Can you work these out from the model? Positions are in its coordinate system, mm. A direction names the side the tool comes from. Coordinates: 2 decimals unless noted, no trailing zeros. Order: outer loops, then holes, each group sorted by start corner. A loop starts at its lowest first (then second) coordinate and runs counter-clockwise, first axis right, second up. Notation, with made-up numbers: M -24.5,60.5 L 31.5,60.5 A31 cw 31.5,84.5 Z; hole C -25,-27.75 d7. An arc over 180 degrees is marked long. Answer as a JSON object with one key per item and string values.
from build123d import *

# Parameters (mm, degrees)
F0_W     = 31.242
F0_H     = 22.86
F0_W_2   = 26.67
F0_H_2   = 68.834
F1_DEPTH = 50.8
F2_R     = 12.7
F3_R     = 12.7
F4_R     = 1.27
F5_R     = 2.54
F6_R     = 2.54
F7_DEPTH = 25.4
F8_DEPTH = 15.24
F9_DEPTH = 22.86


with BuildPart() as f1:
    # F0 (on Top) → F1 (new body)
    with BuildSketch(Plane.XY):
        Polygon((-191.1348653173, 27.6544209014), (-191.1348653173, -124.7455790986), (-64.1348653173, -124.7449096382), (-64.1348653173, 27.6544209014), (-127.6348653138, 53.0544209014), align=None)
        with Locations((-150.1138653173, -100.6154452065)):
            Rectangle(F0_W, F0_H, mode=Mode.SUBTRACT)
        with Locations((-105.1558653173, -100.6154452065)):
            Rectangle(F0_W, F0_H, mode=Mode.SUBTRACT)
        Polygon((-153.0348653138, -51.3395790986), (-127.6348653138, -51.3395790986), (-102.2348653138, -51.3395790986), (-102.2348653138, -79.2795790986), (-153.0348653138, -79.2795790986), align=None, mode=Mode.SUBTRACT)
        Polygon((-154.3048653138, 27.6544209014), (-127.6348653138, 27.6544209014), (-100.9648653138, 27.6544209014), (-100.9648653138, -41.1795790986), (-127.6348653138, -41.1795790986), (-154.3048653138, -41.1795790986), align=None, mode=Mode.SUBTRACT)
        with Locations((-140.9698653138, -6.7625790986)):
            Rectangle(F0_W_2, F0_H_2)
        with Locations((-114.2998653138, -6.7625790986)):
            Rectangle(F0_W_2, F0_H_2)
        with Locations((-150.1138653173, -100.6154452065)):
            Rectangle(F0_W, F0_H)
        with Locations((-105.1558653173, -100.6154452065)):
            Rectangle(F0_W, F0_H)
        Polygon((-102.2348653138, -51.3395790986), (-127.6348653138, -51.3395790986), (-153.0348653138, -51.3395790986), (-153.0348653138, -79.2795790986), (-102.2348653138, -79.2795790986), align=None)
    extrude(amount=-F1_DEPTH)

    # F2
    f2_edges = [f1.edges().sort_by_distance(p)[0] for p in [
        (-64.134865, 27.654421, -25.4),
    ]]
    fillet(f2_edges, radius=F2_R)

    # F3
    f3_edges = [f1.edges().sort_by_distance(p)[0] for p in [
        (-191.134865, 27.654421, -25.4),
    ]]
    fillet(f3_edges, radius=F3_R)

    # F4
    f4_edges = [f1.edges().sort_by_distance(p)[0] for p in [
        (-127.634865, 53.054421, -25.4),
    ]]
    fillet(f4_edges, radius=F4_R)

    # F5
    f5_edges = [f1.edges().sort_by_distance(p)[0] for p in [
        (-191.134865, -124.745579, -25.4),
    ]]
    fillet(f5_edges, radius=F5_R)

    # F6
    f6_edges = [f1.edges().sort_by_distance(p)[0] for p in [
        (-64.134865, -124.74491, -25.4),
    ]]
    fillet(f6_edges, radius=F6_R)

    # F0 (on Top) → F7 (cut)
    with BuildSketch(Plane.XY):
        with Locations((-140.9698653138, -6.7625790986)):
            Rectangle(F0_W_2, F0_H_2)
        with Locations((-114.2998653138, -6.7625790986)):
            Rectangle(F0_W_2, F0_H_2)
    extrude(amount=-F7_DEPTH, mode=Mode.SUBTRACT)

    # F0 (on Top) → F8 (cut)
    with BuildSketch(Plane.XY):
        with Locations((-150.1138653173, -100.6154452065)):
            Rectangle(F0_W, F0_H)
        with Locations((-105.1558653173, -100.6154452065)):
            Rectangle(F0_W, F0_H)
    extrude(amount=-F8_DEPTH, mode=Mode.SUBTRACT)

    # F0 (on Top) → F9 (cut)
    with BuildSketch(Plane.XY):
        Polygon((-102.2348653138, -51.3395790986), (-127.6348653138, -51.3395790986), (-153.0348653138, -51.3395790986), (-153.0348653138, -79.2795790986), (-102.2348653138, -79.2795790986), align=None)
    extrude(amount=-F9_DEPTH, mode=Mode.SUBTRACT)


solid = f1.part
Item 1: I want a section at C-C, the plane z = -5. Write out the boundary of the cut face in (x, y).
Answers follow:
{"outline": "M -191.13,-122.21 A2.54 ccw -188.59,-124.75 L -66.67,-124.74 A2.54 ccw -64.13,-122.2 L -64.13,19.06 A12.7 ccw -72.12,30.85 L -127.16,52.87 A1.27 ccw -128.11,52.87 L -183.15,30.85 A12.7 ccw -191.13,19.06 Z; hole M -165.73,-112.05 L -134.49,-112.05 L -134.49,-89.19 L -165.73,-89.19 Z; hole M -154.3,-41.18 L -100.96,-41.18 L -100.96,27.65 L -154.3,27.65 Z; hole M -153.03,-79.28 L -102.23,-79.28 L -102.23,-51.34 L -153.03,-51.34 Z; hole M -120.78,-112.05 L -89.53,-112.05 L -89.53,-89.19 L -120.78,-89.19 Z"}
Item 2: I want a section at D-D, the plane x = -98.5. Write out the boundary of the cut face in (y, z), plus the area to 3 significant figures.
Answers follow:
{"outline": "M -124.75,-50.8 L 41.4,-50.8 L 41.4,0 L -89.19,0 L -89.19,-15.24 L -112.05,-15.24 L -112.05,0 L -124.75,0 Z", "area": "8,090 mm^2"}
Item 3: I want a section at B-B, the plane y = -57. Write out the boundary of the cut face in (x, z), plus the area to 3 significant figures.
Answers follow:
{"outline": "M -191.13,-50.8 L -64.13,-50.8 L -64.13,0 L -102.23,0 L -102.23,-22.86 L -153.03,-22.86 L -153.03,0 L -191.13,0 Z", "area": "5,290 mm^2"}
Item 4: If we mould it in two halves opening along X, with no side actions, what happens to faces 3 (the flat face through (-191.135, -51, -25)), 4 (the flat face through (-129, -35, -50.8)), 5 (the flat face through (-64.135, -53, -25)), 6 (the flat face through (-128, -6, -25.4))? For each: pulls with the +X half, pulls with the -X half, needs draft (parallel to the pull), parting line crosses it, or undercut.
Answers follow:
{"face 3": "pulls with the -X half", "face 4": "needs draft", "face 5": "pulls with the +X half", "face 6": "undercut"}
Item 5: Which directions (+Z, -Z, +X, -X, +Y, -Y) give clear straight access to the entire face, cutting with the end or side of a thin tool? Please do faces 1 (the flat face through (-157, -35, 0)), 2 (the flat face through (-105, -89.185, -8)).
Answers follow:
{"face 1": "+Z, +X, -X, +Y, -Y", "face 2": "+Z"}
Item 6: Please list where these lines run through material, in increasing order: line 1 (X direction, y = -75, z = -8); line 2 (Z direction, x = -151, y = 18); line 3 (Y direction, x = -110.5, z = -16.5).
Answers follow:
{"line 1": "x = -191.13 to -153.03, -102.23 to -64.13", "line 2": "z = -50.8 to -25.4", "line 3": "y = -124.75 to -79.28, -51.34 to -41.18, 27.65 to 46.2"}
Item 7: I want a section at A-A, the plane z = -33.5. Write out the boundary of the cut face in (x, y).
Answers follow:
{"outline": "M -191.13,-122.21 A2.54 ccw -188.59,-124.75 L -66.67,-124.74 A2.54 ccw -64.13,-122.2 L -64.13,19.06 A12.7 ccw -72.12,30.85 L -127.16,52.87 A1.27 ccw -128.11,52.87 L -183.15,30.85 A12.7 ccw -191.13,19.06 Z"}
Item 8: I'm going to push flat-ended pins straight in: pin 1 (16 mm diameter, centred on x = -123, y = -12, fed in from +Z); pin 2 (5 mm diameter, centred on x = -155, z = -5, fed in from +Y); pin 3 (7.5 mm diameter, centred on x = -105.5, z = -5.5, fed in from +Y). Where does each tip first touch, or does it pass through?
Answers follow:
{"pin 1": "stops at z = -25.4", "pin 2": "stops at y = 43.11", "pin 3": "stops at y = 45.7"}
